from build123d import *

# Parameters (mm, degrees)
BOSS_EXTRUDE1_DEPTH     = 61
CUT_EXTRUDE7_DEPTH      = 69.401456719
CUT_EXTRUDE7_DEPTH_BACK = 69.401456719
CUT_EXTRUDE9_DEPTH      = 69.480850828
CUT_EXTRUDE9_DEPTH_BACK = 69.480850828
SKETCH11_R              = 2.25


with BuildPart() as part:
    # Sketch1 → Boss-Extrude1 (new body)
    with BuildSketch(Plane.XY):
        Polygon((-30.5, -2.244929108), (-30.5, -3.744929108), (30.5, 3.744929108), (30.5, 5.244929108), align=None)
    extrude(amount=BOSS_EXTRUDE1_DEPTH)

    # Sketch7 → Cut-Extrude7 (cut, two sides: drawn at the far end of the back side and taken through both)
    with BuildSketch(Plane(origin=(0, 0, 0), x_dir=(1, 0, 0), z_dir=(0, 1, 0)).offset(-CUT_EXTRUDE7_DEPTH_BACK)):
        with BuildLine():
            Line((9.4e-08, 0), (-30.5, 0))
            Line((-30.5, 0), (-30.5, -30.5))
            ThreePointArc((-30.5, -30.5), (-21.566756793, -8.933243141), (9.4e-08, 0))
        make_face()
        with BuildLine():
            Line((30.5, 0), (9.4e-08, 0))
            ThreePointArc((9.4e-08, 0), (21.566756859, -8.933243207), (30.5, -30.5))
            Line((30.5, -30.5), (30.5, 0))
        make_face()
        with BuildLine():
            Line((30.5, -61), (30.5, -30.5))
            ThreePointArc((30.5, -30.5), (21.566756823, -52.066756829), (-8e-09, -61))
            Line((-8e-09, -61), (30.5, -61))
        make_face()
        with BuildLine():
            ThreePointArc((-8e-09, -61), (-21.566756829, -52.066756823), (-30.5, -30.5))
            Line((-30.5, -30.5), (-30.5, -61))
            Line((-30.5, -61), (-8e-09, -61))
        make_face()
    extrude(amount=CUT_EXTRUDE7_DEPTH + CUT_EXTRUDE7_DEPTH_BACK, mode=Mode.SUBTRACT)

    # Sketch11 → Cut-Extrude9 (cut, two sides: drawn at the far end of the back side and taken through both)
    with BuildSketch(Plane(origin=(-0.181441422, 1.477721795, 0), x_dir=(0.992546151641322, 0.12186934340514832, 0), z_dir=(-0.12186934340514831, 0.9925461516413219, 0)).offset(-CUT_EXTRUDE9_DEPTH_BACK)):
        with Locations(Location((0, -12.5, 0), (0, 0, 180))):
            Circle(SKETCH11_R)
        with Locations(Location((0, -48.5, 0), (0, 0, 180))):
            Circle(SKETCH11_R)
    extrude(amount=CUT_EXTRUDE9_DEPTH + CUT_EXTRUDE9_DEPTH_BACK, mode=Mode.SUBTRACT)


solid = part.part
Read the model definition and answer for the solid it produces. Units are mm, in the model's axes. Coordinates: 2 decimals unless noted, no trailing zeros. Write each loop counter-clockwise with the first axis right and the second up, starting at its lowest first coordinate (ties: lowest second). Pieces come first, ordered by that corner, then holes. Notation, with made-up numbers: (6.5, 52) -> (39.5, 52) arc R9 ccw to (39.5, 69) -> close; hole circle Ø1 at (71.5, 54). An arc over 180 degrees is marked (long way). Return JSON: item names as keys, results as strings.
(1) For a pull along Z with two mould halves and no side action, classify faces 1 (the flat face through (0.427, 1.552, 30.073)), 2 (the cylindrical face through (0.2, 0.76, 50.73)), 3 (the cylindrical face through (0.2, 0.76, 14.73)) as pulls with the +Z half, pulls with the -Z half, needs draft (parallel to the pull), parting line crosses it, or undercut.
Answers below:
{"face 1": "needs draft", "face 2": "undercut", "face 3": "undercut"}
(2) The part is cut by section C-C on x = 12.5. Give the vertices of the cut face in (y, z).
Answers below:
{"outline": "(1.53, 2.68) -> (3.03, 2.68) -> (3.03, 58.32) -> (1.53, 58.32) -> close"}
(3) Consider line 1 along Y through (x, z) = (-5, 10.5); line 2 along Y through (x, z) = (15, 13). Determine where each line is inside the solid, lowest interval first. Write a range as from..to.
Answers below:
{"line 1": "-0.61..0.89", "line 2": "1.84..3.34"}
(4) The part is cut by section A-A on z = 47.5. Give the vertices of the cut face in (x, y), then the cut area to 3 significant figures.
Answers below:
{"outline": "(-25.32, -3.11) -> (-2, -0.25) -> (-2.18, 1.23) -> (-25.32, -1.61) -> close; (1.82, 1.72) -> (2, 0.25) -> (25.32, 3.11) -> (25.32, 4.61) -> close", "area": "70.0 mm^2"}
(5) The part is cut by section B-B on y = -1.5. Give the vertices of the cut face in (x, z), then the cut area to 3 significant figures.
Answers below:
{"outline": "(-24.43, 12.24) arc R30.5 ccw to (-12.22, 2.55) -> (-12.22, 58.45) arc R30.5 ccw to (-24.43, 48.76) -> close", "area": "586 mm^2"}
